Can you work these out from the drawing? Everything is in mm from the part's minimum corner. A direction names the side the tool comes from. Give positions to 0.01 mm unless a question says otherwise; leave off trailing zeros. Write each loop counter-clockwise with the first axis right and the second up, starting at its lowest first coordinate (ties: lowest second). Pieces come first, ordered by that corner, then holes. Notation, with made-up numbers: (24, 46) - (58, 46) arc R27 ccw to (58, 82) - close; hole circle Ø9 at (13.25, -20). An arc over 180 degrees is marked (long way). Use a Markdown table: item, result.
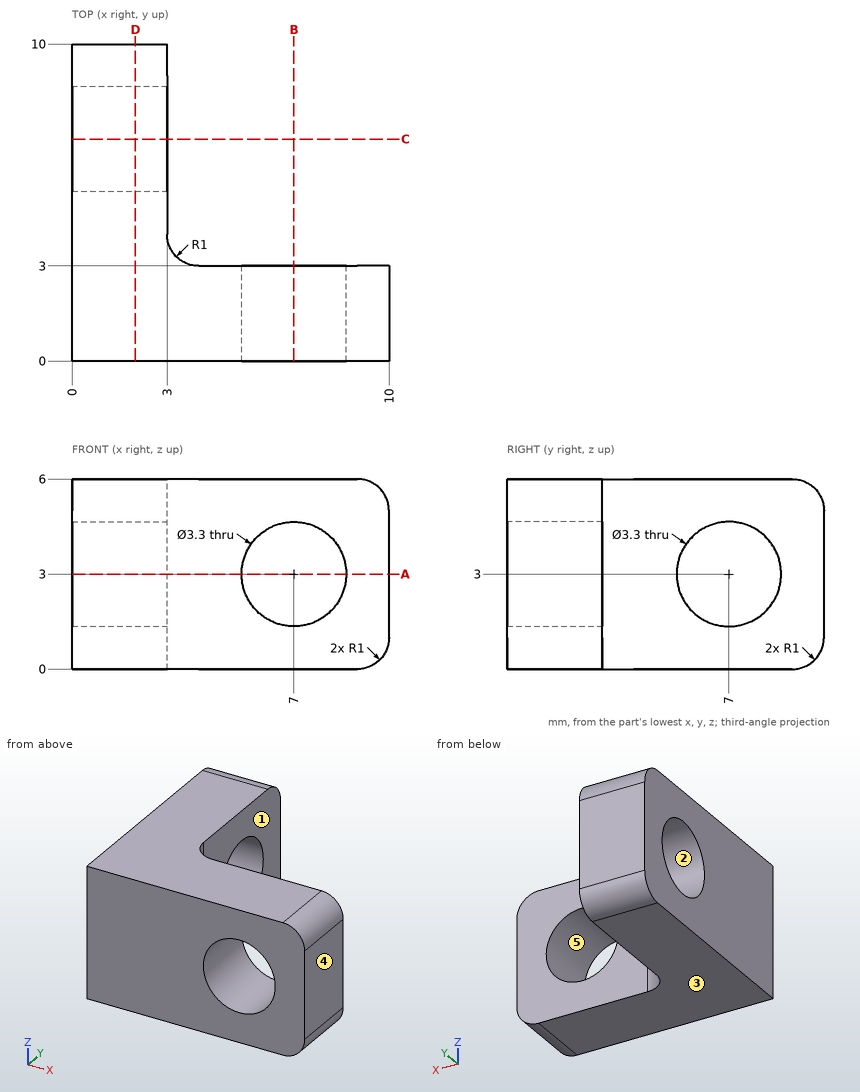
Item 1: Will these pins go through, and if not, where does the flat tip stop? pin 1 Ø1 at (x, z) = (4, 1) entering from +Y; pin 2 Ø1.8 at (x, z) = (6.5, 2) entering from +Y.
Values:
| item | result |
|---|---|
| pin 1 | stops at y = 3.13 |
| pin 2 | stops at y = 3 |
Item 2: If we section it at A-A, the plane z = 3: Write out the boundary of the cut face in (x, y), plus the area to 3 significant figures.
Values:
| item | result |
|---|---|
| outline | (0, 0) - (5.35, 0) - (5.35, 3) - (4, 3) arc R1 cw to (3, 4) - (3, 5.35) - (0, 5.35) - close; (0, 8.65) - (3, 8.65) - (3, 10) - (0, 10) - close; (8.65, 0) - (10, 0) - (10, 3) - (8.65, 3) - close |
| area | 31.4 mm2 |
Item 3: If we section it at D-D, the plane x = 2: Write out the boundary of the cut face in (y, z).
Values:
| item | result |
|---|---|
| outline | (0, 0) - (9, 0) arc R1 ccw to (10, 1) - (10, 5) arc R1 ccw to (9, 6) - (0, 6) - close; hole circle Ø3.3 at (7, 3) |
Item 4: I need wall thicknesses on line 1 along Z through (x, y) = (2.15, 7); line 2 along X through (y, z) = (1.1, 3); line 3 along Y through (x, z) = (5, 3.65). Which ranges of each line are inside material? Lowest first, please. Write a range as [from, to].
Values:
| item | result |
|---|---|
| line 1 | z = [0, 1.35], [4.65, 6] |
| line 2 | x = [0, 5.35], [8.65, 10] |
| line 3 | y = [0, 3] |
Item 5: If we section it at B-B, the plane x = 7: Write out the boundary of the cut face in (y, z), plus the area to 3 significant figures.
Values:
| item | result |
|---|---|
| outline | (0, 0) - (3, 0) - (3, 1.35) - (0, 1.35) - close; (0, 4.65) - (3, 4.65) - (3, 6) - (0, 6) - close |
| area | 8.10 mm2 |
Item 6: For the marked faces 1 and 2, which set-ups out of +Z, -Z, +X, -X, +Y, -Y let a thin tool reach every point of the face, with its end or its side?
Values:
| item | result |
|---|---|
| face 1 | +Z, -Z, +X, +Y |
| face 2 | +X, -X |
Item 7: Thinking about a two-plate mould opening in X: for the marked faces 3, 4 and 5, which applies, +X half, -X half, draft (parallel to the pull), parting line (faces both ways), or undercut?
Values:
| item | result |
|---|---|
| face 3 | draft |
| face 4 | +X half |
| face 5 | undercut |
